from build123d import *

# Parameters (mm, degrees)
BOSS_EXTRUDE1_DEPTH = 2.4
SKETCH2_R           = 32.5
BOSS_EXTRUDE2_DEPTH = 10
SKETCH3_R           = 29
BOSS_EXTRUDE3_DEPTH = 12
BOSS_EXTRUDE3_TAPER = 22.5


with BuildPart() as part:
    # Sweep2: sweep along a path in BasketRing
    with BuildLine(Plane.XY) as sweep2_path:
        Line((44, 0), (273.5, 0))
        ThreePointArc((273.5, 0), (304.612698372, 12.887301628), (317.5, 44))
        Line((317.5, 44), (317.5, 203.5))
        ThreePointArc((317.5, 203.5), (304.612698372, 234.612698372), (273.5, 247.5))
        Line((273.5, 247.5), (44, 247.5))
        ThreePointArc((44, 247.5), (12.887301628, 234.612698372), (0, 203.5))
        Line((0, 203.5), (0, 44))
        ThreePointArc((0, 44), (12.887301628, 12.887301628), (44, 0))
    # ShapeOf Edge → Sweep2 (sweep)
    with BuildSketch(Plane(origin=(44, 0, 0), x_dir=(0, 0, -1), z_dir=(1, 0, 0))):
        Polygon((0, 0), (2.4, 0), (4.8, -2.4), (30.4, -2.4), (30.4, 0), (5.79411255, 0), (2.4, 3.39411255), (2.4, 7), (0, 7), align=None)
    sweep(path=sweep2_path.line)

    # Sketch1 → Boss-Extrude1 (add)
    with BuildSketch(Plane.XY):
        with BuildLine():
            Line((44, 240.5), (273.5, 240.5))
            ThreePointArc((273.5, 240.5), (299.662950904, 229.662950904), (310.5, 203.5))
            Line((310.5, 203.5), (310.5, 44))
            ThreePointArc((310.5, 44), (299.662950904, 17.837049096), (273.5, 7))
            Line((273.5, 7), (44, 7))
            ThreePointArc((44, 7), (17.837049096, 17.837049096), (7, 44))
            Line((7, 44), (7, 203.5))
            ThreePointArc((7, 203.5), (17.837049096, 229.662950904), (44, 240.5))
        make_face()
    extrude(amount=-BOSS_EXTRUDE1_DEPTH)

    # Sketch2 → Boss-Extrude2 (add)
    with BuildSketch(Plane(origin=(0, 0, -2.4), x_dir=(-1, 0, 0), z_dir=(0, 0, -1))):
        with Locations((-158.75, 123.75)):
            Circle(SKETCH2_R)
    extrude(amount=BOSS_EXTRUDE2_DEPTH)

    # Sketch3 → Boss-Extrude3 (add)
    with BuildSketch(Plane(origin=(0, 0, -12.4), x_dir=(-1, 0, 0), z_dir=(0, 0, -1))):
        with Locations((-158.75, 123.75)):
            Circle(SKETCH3_R)
    extrude(amount=BOSS_EXTRUDE3_DEPTH, taper=BOSS_EXTRUDE3_TAPER)


solid = part.part
Check sheet for the modelled part. Datum: model origin and axes. Units: mm. A direction names the side the tool comes from. Round coordinates to 2 decimals unless told otherwise and drop trailing zeros. Order: outer loops, then holes, each group sorted by start corner. A loop starts at its lowest first (then second) coordinate and runs counter-clockwise, first axis right, second up. Notation, with made-up numbers: M 26,-2.75 L 56,-2.75 A30 cw 56,34.25 Z; hole C -27,62 d8. An arc over 180 degrees is marked long. One line per item, written item: value. Start each with the question number.
1. Release check for a two-part mould opening along Y. For faces 1 (the cylindrical face through (184.54, 103.97, -7.33)), 2 (the conical face through (135.6, 131.04, -23.82)), 3 (the conical face through (12.44, 13.13, -2.55)), 4 (the flat face through (157, 249.9, -17)) record: released by +Y, released by -Y, zero draft, split by the parting line, or undercut.
2. Scan lines: line 1 along Y through (x, z) = (233, -8.5); line 2 along X through (y, z) = (178.5, -15.5); line 3 along X through (y, z) = (151.5, -3.5). Record each from-to range of solid material in increasing order.
3. Gauge pin test, flat ends, axial feed: P1, Ø1, axis at x = 277.5, z = -25, coming from the +Y side; P2, Ø1.2, axis at x = 158.5, z = -1.5, coming from the -Y side; P3, Ø24, axis at x = 152.5, y = 132.5, coming from the -Z side. Record the tip position at first contact, or that the pin passes through.
4. Section check C-C on y = 177.5. Enter the section's corners in (x, z).
5. Section check D-D on x = 158.75. Enter the section's corners in (y, z), and give its area (3 significant figures).
6. Access from +Z, -Z, +X, -X, +Y, -Y to the whole of each face (thin tool, end or side, straight path). Record for faces 5 (the cylindrical face through (304.95, 234.27, -1.22)), 6 (the conical face through (302.01, 14.86, -2.56)), 7 (the cylindrical face through (13.23, 234.95, -1.22)).
7. Section check A-A on z = -19. Enter the section's corners in (x, y), and give its area (3 significant figures).
8. Section check B-B on x = 256. Enter the section's corners in (y, z).
Results found:
1. face 1: undercut
1. face 2: undercut
1. face 3: released by -Y
1. face 4: released by +Y
2. line 1: -2.4 to 0, 247.5 to 249.9
2. line 2: -2.4 to 0, 317.5 to 319.9
2. line 3: -1.1 to 2.29, 141.83 to 175.67, 315.21 to 318.6
3. P1: y = 249.77
3. P2: y = 0
3. P3: z = -24.4
4. outline: M -2.4,-30.4 L 0,-30.4 L 0,-5.79 L 3.39,-2.4 L 314.11,-2.4 L 317.5,-5.79 L 317.5,-30.4 L 319.9,-30.4 L 319.9,-4.8 L 317.5,-2.4 L 317.5,0 L 0,0 L 0,-2.4 L -2.4,-4.8 Z
5. outline: M -2.4,-30.4 L 0,-30.4 L 0,-5.79 L 3.39,-2.4 L 91.25,-2.4 L 91.25,-12.4 L 94.75,-12.4 L 99.72,-24.4 L 147.78,-24.4 L 152.75,-12.4 L 156.25,-12.4 L 156.25,-2.4 L 244.11,-2.4 L 247.5,-5.79 L 247.5,-30.4 L 249.9,-30.4 L 249.9,-4.8 L 247.5,-2.4 L 247.5,0 L 0,0 L 0,-2.4 L -2.4,-4.8 Z
5. area: 2,020 mm^2
6. face 5: +Z, +X, +Y
6. face 6: -Z
6. face 7: +Z, -X, +Y
7. outline: M -2.4,44 A46.4 ccw 44,-2.4 L 273.5,-2.4 A46.4 ccw 319.9,44 L 319.9,203.5 A46.4 ccw 273.5,249.9 L 44,249.9 A46.4 ccw -2.4,203.5 Z; C 158.75,123.75 d52.53; hole M 0,44 A44 ccw 44,0 L 273.5,0 A44 ccw 317.5,44 L 317.5,203.5 A44 ccw 273.5,247.5 L 44,247.5 A44 ccw 0,203.5 Z
7. area: 4,720 mm^2
8. outline: M -2.4,-30.4 L 0,-30.4 L 0,-5.79 L 3.39,-2.4 L 244.11,-2.4 L 247.5,-5.79 L 247.5,-30.4 L 249.9,-30.4 L 249.9,-4.8 L 247.5,-2.4 L 247.5,0 L 0,0 L 0,-2.4 L -2.4,-4.8 Z
